from build123d import *

# Parameters (mm, degrees)
SKETCH_1_W      = 89
SKETCH_1_H      = 52
EXTRUDE_1_DEPTH = 35
EXTRUDE_2_DEPTH = 0.5


with BuildPart() as part:
    # Эскиз1 → Бобышка-Вытянуть1 (new body)
    with BuildSketch(Plane(origin=(0, 0, 0), x_dir=(1, 0, 0), z_dir=(0, 1, 0))):
        with Locations((44.5, 26)):
            Rectangle(SKETCH_1_W, SKETCH_1_H)
    extrude(amount=EXTRUDE_1_DEPTH)

    # Эскиз2 → Бобышка-Вытянуть2 (add)
    with BuildSketch(Plane.XZ):
        with BuildLine():
            Line((-10.5, -37), (13.5, -37))
            Line((13.5, -37), (13.5, -15))
            Line((13.5, -15), (-10.5, -15))
            ThreePointArc((-10.5, -15), (-12.621320344, -15.878679656), (-13.5, -18))
            Line((-13.5, -18), (-13.5, -34))
            ThreePointArc((-13.5, -34), (-12.621320344, -36.121320344), (-10.5, -37))
        make_face()
        with BuildLine():
            Line((-5, -20.5), (-5, -23.763932023))
            ThreePointArc((-5, -23.763932023), (-4, -26), (-5, -28.236067977))
            Line((-5, -28.236067977), (-5, -31.5))
            ThreePointArc((-5, -31.5), (-7, -33.5), (-9, -31.5))
            Line((-9, -31.5), (-9, -28.236067977))
            ThreePointArc((-9, -28.236067977), (-10, -26), (-9, -23.763932023))
            Line((-9, -23.763932023), (-9, -20.5))
            ThreePointArc((-9, -20.5), (-7, -18.5), (-5, -20.5))
        make_face(mode=Mode.SUBTRACT)
        with BuildLine():
            Line((75.5, -37), (75.5, -15))
            Line((75.5, -15), (99.5, -15))
            ThreePointArc((99.5, -15), (101.621320344, -15.878679656), (102.5, -18))
            Line((102.5, -18), (102.5, -34))
            ThreePointArc((102.5, -34), (101.621320344, -36.121320344), (99.5, -37))
            Line((99.5, -37), (75.5, -37))
        make_face()
        with BuildLine():
            Line((98, -28.236067977), (98, -31.5))
            ThreePointArc((98, -31.5), (96, -33.5), (94, -31.5))
            Line((94, -31.5), (94, -28.236067977))
            ThreePointArc((94, -28.236067977), (93, -26), (94, -23.763932022))
            Line((94, -23.763932022), (94, -20.5))
            ThreePointArc((94, -20.5), (96, -18.5), (98, -20.5))
            Line((98, -20.5), (98, -23.763932022))
            ThreePointArc((98, -23.763932022), (99, -26), (98, -28.236067977))
        make_face(mode=Mode.SUBTRACT)
    extrude(amount=-EXTRUDE_2_DEPTH)


solid = part.part
Here's how the part is built. I have some questions about the finished solid (model axes, mm). A direction names the side the tool comes from. Coordinates: 2 decimals unless noted, no trailing zeros. Write each loop counter-clockwise with the first axis right and the second up, starting at its lowest first coordinate (ties: lowest second). Pieces come first, ordered by that corner, then holes.
Item 1: I want a section at A-A on x = -7. Write out the boundary of the cut face in (y, z).
Item 2: If we mould it in two halves opening along X, with no side actions, what happens to faces 1 (the cylindrical face through (101.6, 0.25, -15.86)), 2 (the cylindrical face through (-7, 0.2, -33.5)), 3 (the flat face through (44, 17, 0))? For each: +X half, -X half, draft (parallel to the pull), parting line (faces both ways), or undercut.
Item 3: I want a section at B-B on z = -35.5. Write out the boundary of the cut face in (x, y), and give its area (3 significant figures).
Item 4: If I drill on line 1 (X direction, y = 17.5, z = -47.5); line 2 (Y direction, x = -4, z = -17), over which ranges is the centre line in solid material (lowest first)?
Item 5: I want a section at C-C on y = 15.5. Write out the boundary of the cut face in (x, z), and give its area (3 significant figures).
Item 6: Will these pins go through, and if not, where does the flat tip stop? pin 1 (10.5 mm diameter, centred on y = 14, z = -32.5, fed in from -X); pin 2 (17.5 mm diameter, centred on y = 11.5, z = -22, fed in from +X).
Item 7: I want a section at D-D on z = -12. Write out the boundary of the cut face in (x, y), and give its area (4 significant figures).
Item 8: On a 3-axis mill with a long thin cutter (end or side, diameter ignored), from which of +Z, -Z, +X, -X, +Y, -Y can I reach the whole of each face in a straight line? I mean faces 4 (the flat face through (92.8, 0.5, -25.8)), 5 (the flat face through (-3.8, 0.5, -25.8)), 6 (the cylindrical face through (96, 0.2, -18.5)), 7 (the flat face through (44, 17, -52)). Say none if no direction works.
Findings below:
1. outline: (0, -37) - (0.5, -37) - (0.5, -33.5) - (0, -33.5) - close; (0, -18.5) - (0.5, -18.5) - (0.5, -15) - (0, -15) - close
2. face 1: +X half
2. face 2: undercut
2. face 3: draft
3. outline: (-13.1, 0) - (102.1, 0) - (102.1, 0.5) - (89, 0.5) - (89, 35) - (0, 35) - (0, 0.5) - (-13.1, 0.5) - close
3. area: 3,130 mm2
4. line 1: x = 0 to 89
4. line 2: y = 0 to 0.5
5. outline: (0, -52) - (89, -52) - (89, 0) - (0, 0) - close
5. area: 4,630 mm2
6. pin 1: stops at x = 0
6. pin 2: stops at x = 89
7. outline: (0, 0) - (89, 0) - (89, 35) - (0, 35) - close
7. area: 3,115 mm2
8. face 4: +Z, -Z, +X, +Y
8. face 5: +Z, -Z, -X, +Y
8. face 6: +Y, -Y
8. face 7: -Z, +X, -X, +Y, -Y
